```python
from build123d import *

# Parameters (mm, degrees)
SKETCH_1_R               = 25
EXTRUDE_1_DEPTH          = 10
CUT_EXTRUDE_1_DEPTH      = 37.742346142
PATTERN_CIRCULAR_1_COUNT = 20
CUT_EXTRUDE_2_DEPTH      = 37.334492668
PATTERN_CIRCULAR_2_COUNT = 20


with BuildPart() as part:
    # 草图1 → 凸台-拉伸1 (new body)
    with BuildSketch(Plane(origin=(0, 0, 0), x_dir=(1, 0, 0), z_dir=(0, 1, 0))):
        with Locations(Location((0, 0, 0), (0, 0, 270))):
            Circle(SKETCH_1_R)
        with BuildLine():
            Line((5.788177086, 3.936623684), (10.900331071, 3.936623684))
            Line((10.900331071, 3.936623684), (10.900331071, -3.936623684))
            Line((10.900331071, -3.936623684), (5.788177086, -3.936623684))
            ThreePointArc((5.788177086, -3.936623684), (-7, 0), (5.788177086, 3.936623684))
        make_face(mode=Mode.SUBTRACT)
    extrude(amount=EXTRUDE_1_DEPTH)

    # 草图2 → 切除-拉伸1 (cut, symmetric)
    with BuildSketch(Plane(origin=(0, 10, 0), x_dir=(1, 0, 0), z_dir=(0, 1, 0))):
        Polygon((-1.89299605, 16.850353612), (1.89299605, 16.850353612), (1.89299605, 19.294888065), (6.011008964, 30.60903556), (-6.011008964, 30.60903556), (-1.89299605, 19.294888065), align=None)
    cut_extrude_1 = extrude(amount=CUT_EXTRUDE_1_DEPTH, both=True, mode=Mode.SUBTRACT)

    # 阵列(圆周)1: 切除-拉伸1 ×20 about axis
    pattern_circular_1_axis = Axis((0, 0, 0), (0, 1, 0))
    for i in range(1, PATTERN_CIRCULAR_1_COUNT):
        add(cut_extrude_1.rotate(pattern_circular_1_axis, i * 360 / PATTERN_CIRCULAR_1_COUNT), mode=Mode.SUBTRACT)

    # 草图4 → 切除-拉伸2 (cut, symmetric)
    with BuildSketch(Plane(origin=(0, 0, 0), x_dir=(1, 0, 0), z_dir=(0, 1, 0))):
        Polygon((-5.064708137, 21.29319636), (-2.398933181, 21.715413634), (-3.215562642, 26.871409132), (-6.421705824, 26.363605939), align=None)
    cut_extrude_2 = extrude(amount=CUT_EXTRUDE_2_DEPTH, both=True, mode=Mode.SUBTRACT)

    # 阵列(圆周)2: 切除-拉伸2 ×20 about axis
    pattern_circular_2_axis = Axis((0, 0, 0), (0, 1, 0))
    for i in range(1, PATTERN_CIRCULAR_2_COUNT):
        add(cut_extrude_2.rotate(pattern_circular_2_axis, i * 360 / PATTERN_CIRCULAR_2_COUNT), mode=Mode.SUBTRACT)


solid = part.part
```
Could you check a few things on this model? Use its own coordinates, in mm. A direction names the side the tool comes from. Round coordinates to 2 decimals unless told otherwise and drop trailing zeros. Loops run counter-clockwise (first coordinate to the right, second up) from the corner with the lowest first, then second, coordinate; pieces in that order, holes last. Notation, with made-up numbers: (44, 47) - (95, 47) arc R16 ccw to (95, 61) - close; hole circle Ø11 at (75.25, -11.75). An arc over 180 degrees is marked (long way). Answer in a Markdown table with one row per item. Add a question column.
(1) I'm going to push flat-ended pins straight in: pin 1 (2.5 mm diameter, centred on x = 18.5, y = 4, fed in from +Z); pin 2 (0.7 mm diameter, centred on x = -18.5, y = 6, fed in from +Z); pin 3 (1.2 mm diameter, centred on y = 4, z = -18.5, fed in from -X). Where does each tip first touch, or does it pass through?
(2) If we section it at C-C (x = -12): Please give me the cut outline in (y, z), plus the area to 3 significant figures.
(3) If we section it at B-B (x = 0): Please give me the cut outline in (y, z).
(4) I need wall thicknesses on line 1 along Z through (x, y) = (0, 4.5); line 2 along X through (y, z) = (4.5, 0); line 3 along X through (y, z) = (6, -13.5). Which ranges of each line are inside material? Lowest first, please.
(5) If we mould it in two halves opening along Z, with no side actions, what happens to faces 5 (the face through (1.893, 5, 18)), 6 (the face through (-18, 5, 1.893)), 7 (the face through (-19.44, 5.07, 9.92))? For each: pulls with the +Z half, pulls with the -Z half, needs draft (parallel to the pull), parting line crosses it, or undercut.
(6) If we section it at A-A (z = 0): Please give me the cut outline in (x, y).
(7) For faces 1 (the face through (18.743, 5.07, 8.526)), 2 (the face through (-10.15, 5.07, -17.91)), 3 (the face through (-17.95, 5.07, -10.16)), 4 (the face through (9.101, 5.07, -15.748)), which set-ups out of +Z, -Z, +X, -X, +Y, -Y let a thin tool reach every point of the face, with its end or its side?
Model answer:
| question | item | result |
|---|---|---|
| 1 | pin 1 | stops at z = 10.5 |
| 1 | pin 2 | stops at z = 10.42 |
| 1 | pin 3 | stops at x = -10.49 |
| 2 | outline | (0, -13.3) - (10, -13.3) - (10, 13.3) - (0, 13.3) - close |
| 2 | area | 266 mm² |
| 3 | outline | (0, -16.85) - (10, -16.85) - (10, -7) - (0, -7) - close; (0, 7) - (10, 7) - (10, 16.85) - (0, 16.85) - close |
| 4 | line 1 | z = -16.85 to -7, 7 to 16.85 |
| 4 | line 2 | x = -16.85 to -7, 10.9 to 16.85 |
| 4 | line 3 | x = -14.92 to -12.15, -10.09 to 10.09, 12.15 to 14.92 |
| 5 | face 5 | needs draft |
| 5 | face 6 | undercut |
| 5 | face 7 | pulls with the +Z half |
| 6 | outline | (-16.85, 0) - (-7, 0) - (-7, 10) - (-16.85, 10) - close; (10.9, 0) - (16.85, 0) - (16.85, 10) - (10.9, 10) - close |
| 7 | face 1 | +X, +Y, -Y |
| 7 | face 2 | -X, +Y, -Y |
| 7 | face 3 | -Z, +Y, -Y |
| 7 | face 4 | +Y, -Y |
